from build123d import *

# Parameters (mm, degrees)
F0_W     = 300
F0_H     = 200
F1_DEPTH = 10
F2_R     = 10
F3_DEPTH = 200
F4_R     = 10
F5_W     = 20
F5_H     = 1
F6_DEPTH = 21
F9_DEPTH = 100
F10_R    = 9.99999


# Not quite as in the source:
# - a fillet or chamfer is up to 0.001 mm smaller than in the source, because OpenCascade refuses the exact size


with BuildPart() as f1:
    # F0 (on Top) → F1 (new body)
    with BuildSketch(Plane.XY):
        with Locations((-5.7550377341, -0.1439023763)):
            Rectangle(F0_W, F0_H)
    extrude(amount=F1_DEPTH)

    # F2 (on face) → F3 (join)
    with BuildSketch(Plane(origin=(0, 0, 0), x_dir=(1, 0, 0), z_dir=(0, 0, -1))):
        with Locations((-125.7550377341, 70.1439023763)):
            Circle(F2_R)
        with Locations((-125.7550377341, -44.8560976237)):
            Circle(F2_R)
        with Locations((114.2449622659, 45.1439023763)):
            Circle(F2_R)
        with Locations((114.2449622659, -69.8560976237)):
            Circle(F2_R)
    extrude(amount=F3_DEPTH)

    # F4
    f4_edges = [f1.edges().sort_by_distance(p)[0] for p in [
        (-135.755038, -70.143902, -200),
        (-135.755038, 44.856098, -200),
        (104.244962, -45.143902, -200),
        (104.244962, 69.856098, -200),
    ]]
    fillet(f4_edges, radius=F4_R)

    # F5 (on face) → F6 (join)
    with BuildSketch(Plane(origin=(0, 0, 0), x_dir=(1, 0, 0), z_dir=(0, 0, -1))):
        with Locations((-125.7550377341, 59.5939023763)):
            Rectangle(F5_W, F5_H)
        with Locations((-125.7550377341, -34.3060976237)):
            Rectangle(F5_W, F5_H)
        with Locations((114.2449622659, -59.3060976237)):
            Rectangle(F5_W, F5_H)
        with Locations((114.2449622659, 34.5939023763)):
            Rectangle(F5_W, F5_H)
    extrude(amount=F6_DEPTH)

    # F7 (on face) + F8 (on face) → F9 (join)
    with BuildSketch(Plane(origin=(0, -59.0939023763, 0), x_dir=(-1, 0, 0), z_dir=(0, 1, 0))):
        with BuildLine():
            ThreePointArc((125.755037734, -21), (132.8261055459, -18.0710678119), (135.7550377341, -11))
            ThreePointArc((135.7550377341, -11), (125.7550377341, -1), (115.7550377341, -11))
            ThreePointArc((115.7550377341, -11), (118.6839699222, -18.0710678119), (125.755037734, -21))
        make_face()
    with BuildSketch(Plane(origin=(0, -34.0939023763, 0), x_dir=(-1, 0, 0), z_dir=(0, 1, 0))):
        with BuildLine():
            ThreePointArc((-114.244962266, -21), (-107.1738944541, -18.0710678119), (-104.2449622659, -11))
            ThreePointArc((-104.2449622659, -11), (-114.2449622659, -1), (-124.2449622659, -11))
            ThreePointArc((-124.2449622659, -11), (-121.3160300778, -18.0710678119), (-114.244962266, -21))
        make_face()
    extrude(amount=F9_DEPTH)

    # F10 (radius 10 in the source; OpenCascade refuses exactly that, so slightly less here)
    f10_edges = [f1.edges().sort_by_distance(p)[0] for p in [
        (-155.755038, -0.143902, 10),
        (-5.755038, 99.856098, 10),
        (144.244962, -0.143902, 10),
        (-5.755038, -100.143902, 10),
    ]]
    fillet(f10_edges, radius=F10_R)


solid = f1.part
Here's how the part is built. I have some questions about the finished solid (model axes, mm). A direction names the side the tool comes from. Give positions to 0.01 mm unless a question says otherwise; leave off trailing zeros. Order: outer loops, then holes, each group sorted by start corner. A loop starts at its lowest first (then second) coordinate and runs counter-clockwise, first axis right, second up. Notation, with made-up numbers: (9.25, 74.5) -> (45.25, 74.5) arc R28 ccw to (45.25, 101.5) -> close; hole circle Ø6 at (3, 50). An arc over 180 degrees is marked (long way). Use a Markdown table: item, result. Add a question column.
Item 1: Will these pins go through, and if not, where does the flat tip stop? pin 1 (5 mm diameter, centred on x = -123, z = -16.5, fed in from +Y); pin 2 (1 mm diameter, centred on x = 30.5, y = -6.5, fed in from -Z); pin 3 (11 mm diameter, centred on x = 110, z = -16, fed in from +Y).
Item 2: Imagine slicing it at D-D on z = -48. Please give me the cut outline in (x, y).
Item 3: I need wall thicknesses on line 1 (Z direction, x = -40.5, y = 24); line 2 (Y direction, x = 117, z = -3); line 3 (Y direction, x = 118, z = -36). Which ranges of each line are inside material? Lowest first, please.
Item 4: Imagine slicing it at A-A on y = 28. Give the number of separate pieces and of enclosed holes in the cut face, plus the area to 3 significant figures.
Item 5: If we mould it in two halves opening along Z, with no side actions, what happens to faces 1 (the face through (114.2, -34.094, -0.6)), 2 (the face through (-128, 34.806, -1)), 3 (the face through (-118, -59.094, -19)), 4 (the face through (-152.903, 1.256, 6.993))? For each: pulls with the +Z half, pulls with the -Z half, needs draft (parallel to the pull), parting line crosses it, or undercut.
Item 6: For faces 5 (the face through (106, 58.806, -19)), 6 (the face through (122, 58.806, -19)), 7 (the face through (106, -34.094, -19)), 8 (the face through (141.393, 1.256, 6.993)), which set-ups out of +Z, -Z, +X, -X, +Y, -Y let a thin tool reach every point of the face, with its end or its side?
Data:
| question | item | result |
|---|---|---|
| 1 | pin 1 | stops at y = 54.85 |
| 1 | pin 2 | stops at z = 0 |
| 1 | pin 3 | stops at y = 79.86 |
| 2 | outline | circle Ø20 at (-125.76, -70.14); circle Ø20 at (-125.76, 44.86); circle Ø20 at (114.24, -45.14); circle Ø20 at (114.24, 69.86) |
| 3 | line 1 | z = 0 to 10 |
| 3 | line 2 | y = -54.76 to -35.53, -35.09 to 79.47 |
| 3 | line 3 | y = -54.41 to -35.88, 60.59 to 79.12 |
| 4 | separate pieces | 3 |
| 4 | enclosed holes | 0 |
| 4 | area | 3,590 mm² |
| 5 | face 1 | undercut |
| 5 | face 2 | undercut |
| 5 | face 3 | needs draft |
| 5 | face 4 | pulls with the +Z half |
| 6 | face 5 | -Z, -X |
| 6 | face 6 | -Z, +X |
| 6 | face 7 | -Z |
| 6 | face 8 | +Z, +X, +Y, -Y |
